```python
from build123d import *

# Parameters (mm, degrees)
SALIENTE_EXTRUIR1_DEPTH = 50
CROQUIS2_R              = 3
CORTAR_EXTRUIR1_DEPTH   = 50


with BuildPart() as part:
    # Croquis1 → Saliente-Extruir1 (new body)
    with BuildSketch(Plane(origin=(0, 0, 0), x_dir=(0, 0, -1), z_dir=(1, 0, 0))):
        with BuildLine():
            Line((1.870828693, -3.25), (24.31662479, -3.25))
            Line((24.31662479, -3.25), (24.31662479, -1.75))
            Line((24.31662479, -1.75), (3.31662479, -1.75))
            ThreePointArc((3.31662479, -1.75), (-2.699984891, 2.602418411), (1.870828693, -3.25))
        make_face()
    extrude(amount=SALIENTE_EXTRUIR1_DEPTH)

    # Croquis2 → Cortar-Extruir1 (cut)
    with BuildSketch(Plane(origin=(0, -1.75, 0), x_dir=(1, 0, 0), z_dir=(0, 1, 0))):
        with Locations(Location((10, 14.31662479, 0), (0, 0, 270))):
            Circle(CROQUIS2_R)
        with Locations(Location((40, 14.31662479, 0), (0, 0, 270))):
            Circle(CROQUIS2_R)
    extrude(amount=-CORTAR_EXTRUIR1_DEPTH, mode=Mode.SUBTRACT)


solid = part.part
```
For this review, take the finished solid that the model builds, in its own axes (mm). A direction names the side the tool comes from. Round coordinates to 2 decimals unless told otherwise and drop trailing zeros. Order: outer loops, then holes, each group sorted by start corner. A loop starts at its lowest first (then second) coordinate and runs counter-clockwise, first axis right, second up. Notation, with made-up numbers: (83.5, 4) -> (130.5, 4) arc R20 cw to (130.5, 34) -> close; hole circle Ø9 at (-2.75, 64.5). An arc over 180 degrees is marked (long way). Use a Markdown table: item, result.
Item 1: For pin 1 (10.5 mm diameter, centred on x = 21, z = -14.5, fed in from +Y); pin 2 (12 mm diameter, centred on x = 12, z = -8, fed in from +Y); pin 3 (8 mm diameter, centred on x = 43, z = -9.5, fed in from -Y); pin 4 (8 mm diameter, centred on x = 33, z = -0.5, fed in from +Y), all flat-tipped, find the tip position at first contact; note any pin that passes through.
Resolved:
| item | result |
|---|---|
| pin 1 | stops at y = -1.75 |
| pin 2 | stops at y = 3.17 |
| pin 3 | stops at y = -3.25 |
| pin 4 | stops at y = 3.75 |
Item 2: For line 1 along Y through (x, z) = (32, -21); line 2 along Z through (x, y) = (21, 2.5), list the stretches that pass through material, from the lowest coordinate up. Write a range as [from, to].
Resolved:
| item | result |
|---|---|
| line 1 | y = [-3.25, -1.75] |
| line 2 | z = [-2.8, 2.8] |
Item 3: Take a section at B-B (z = -21.5). State the section outline as (x, y) points, plus the area to 3 significant figures.
Resolved:
| item | result |
|---|---|
| outline | (0, -3.25) -> (50, -3.25) -> (50, -1.75) -> (0, -1.75) -> close |
| area | 75.0 mm² |
Item 4: Draft analysis for pull direction Z (two halves, no side actions). For faces 3 (the cylindrical face through (10.132, -2.49, -17.314)), 4 (the flat face through (0, -2, -6)), 5 (the flat face through (25, -3, -24.317)), state which applies: +Z half, -Z half, draft (parallel to the pull), parting line (faces both ways), or undercut.
Resolved:
| item | result |
|---|---|
| face 3 | undercut |
| face 4 | draft |
| face 5 | -Z half |
Item 5: Take a section at C-C (x = 27). State the section outline as (y, z) points, plus the area to 3 significant figures.
Resolved:
| item | result |
|---|---|
| outline | (-3.25, -24.32) -> (-1.75, -24.32) -> (-1.75, -3.32) arc R3.75 ccw (long way) to (-3.25, -1.87) -> close |
| area | 76.6 mm² |
Item 6: Machinability: for faces 1 (the flat face through (50, -2, -6)), 2 (the flat face through (25, -3.25, -13)), which of the approach directions +Z, -Z, +X, -X, +Y, -Y give a long, thin tool a straight path to every point of the face, cutting with its end or side? Answer none if there is none.
Resolved:
| item | result |
|---|---|
| face 1 | +Z, -Z, +X, +Y, -Y |
| face 2 | -Z, +X, -X, -Y |
Item 7: Take a section at A-A (x = 10). State the section outline as (y, z) points, plus the area to 3 significant figures.
Resolved:
| item | result |
|---|---|
| outline | (-3.25, -24.32) -> (-1.75, -24.32) -> (-1.75, -17.32) -> (-3.25, -17.32) -> close; (-3.25, -11.32) -> (-1.75, -11.32) -> (-1.75, -3.32) arc R3.75 ccw (long way) to (-3.25, -1.87) -> close |
| area | 67.6 mm² |
